Check sheet for the drawn part. Datum: minimum x, y, z corner. Units: mm. A direction names the side the tool comes from. Coordinates: 2 decimals unless noted, no trailing zeros. Loops run counter-clockwise (first coordinate to the right, second up) from the corner with the lowest first, then second, coordinate; pieces in that order, holes last.
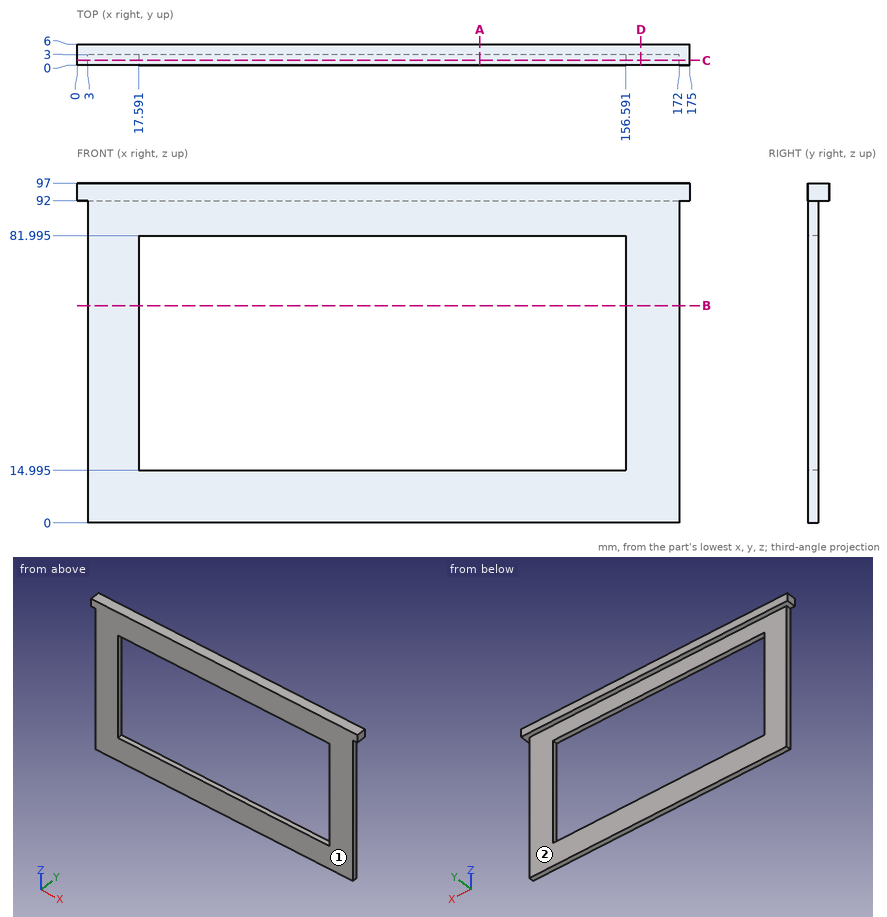
1) Section check D-D on x = 161. Enter the section's corners in (y, z), plus the area to 3 significant figures.
Answer sheet:
outline: (0, 0) - (3, 0) - (3, 92) - (6, 92) - (6, 97) - (0, 97) - close
area: 306 mm2
2) Section check C-C on y = 1.3. Enter the section's corners in (x, z) (1 decimal).
Answer sheet:
outline: (0, 92) - (3, 92) - (3, 0) - (172, 0) - (172, 92) - (175, 92) - (175, 97) - (0, 97) - close; hole (17.6, 15) - (156.6, 15) - (156.6, 82) - (17.6, 82) - close
3) Depth check by flat-ended pin: pin 1 (3 mm diameter, centred on y = 0.5, z = 10, fed in from +X); pin 2 (1.5 mm diameter, centred on x = 130, y = 5, fed in from -Z); pin 3 (2 mm diameter, centred on y = 2.5, z = 21.5, fed in from -X). Enter the tip coordinate at first touch or a pass-through.
Answer sheet:
pin 1: stops at x = 172
pin 2: stops at z = 92
pin 3: stops at x = 3
4) Scan lines: line 1 (X direction, y = 1.9, z = 53); line 2 (Z direction, x = 117.5, y = 2.2) (1 decimal); line 3 (Z direction, x = 74.5, y = 5.2). Record each from-to range of solid material in increasing order.
Answer sheet:
line 1: x = 3 to 17.59, 156.59 to 172
line 2: z = 0 to 15, 82 to 97
line 3: z = 92 to 97
5) Set-up check for the marked faces 1 and 2: record each of +Z, -Z, +X, -X, +Y, -Y from which the full face is reachable in a straight line by a thin tool's end or side.
Answer sheet:
face 1: +Z, -Z, +X, -X, -Y
face 2: -Z, +X, -X, +Y
6) Section check A-A on x = 115. Enter the section's corners in (y, z) (1 decimal).
Answer sheet:
outline: (0, 0) - (3, 0) - (3, 15) - (0, 15) - close; (0, 82) - (3, 82) - (3, 92) - (6, 92) - (6, 97) - (0, 97) - close
7) Section check B-B on z = 62. Enter the section's corners in (x, y).
Answer sheet:
outline: (3, 0) - (17.59, 0) - (17.59, 3) - (3, 3) - close; (156.59, 0) - (172, 0) - (172, 3) - (156.59, 3) - close
